Here's how the part is built. I have some questions about the finished solid (model axes, mm). Face numbers are marked on the shaded views. A direction names the side the tool comes from. Coordinates: 2 decimals unless noted, no trailing zeros. Write each loop counter-clockwise with the first axis right and the second up, starting at its lowest first coordinate (ties: lowest second). Pieces come first, ordered by that corner, then holes.
Item 1: If I drill on line 1 (Y direction, x = 17.2, z = 0); line 2 (Y direction, x = 0, z = -30.25) (3 decimals), over which ranges is the centre line in solid material (lowest first)?
Item 2: If we section it at A-A (z = 0): Count the separate pieces of the cut face and the enclosed holes in it, then the cut area to 3 significant figures.
Item 3: If we section it at B-B (x = 0): Please give me the cut outline in (y, z) (3 decimals), then the cut area to 3 significant figures.
Item 4: For the marked faces 4, 5 and 6, which set-ups out of +Z, -Z, +X, -X, +Y, -Y let a thin tool reach every point of the face, with its end or its side?
Item 5: I'm going to push flat-ended pins straight in: pin 1 Ø8 at (x, z) = (14, -14) entering from -Y; pin 2 Ø12 at (y, z) = (9, -8) entering from -X; pin 3 Ø7.5 at (x, y) = (-0.5, -9) entering from +Z; pin 4 Ø5 at (x, z) = (14.5, -6) entering from +Y. Where does each tip first touch, or does it pass through?
Item 6: We'd pull the mould along Z, two halves only. Please class the marked faces 1, 2 and 3: +Z half, -Z half, draft (parallel to the pull), parting line (faces both ways), or undercut.
from build123d import *

# Parameters (mm, degrees)
BOSS_EXTRUDE1_DEPTH             = 10
CUT_EXTRUDE1_DEPTH              = 46.82575695
CUT_EXTRUDE1_DEPTH_BACK         = 46.82575695
SKETCH2_R                       = 7.5
SKETCH3_R                       = 12.7
SKETCH3_R_2                     = 9.525
BOSS_EXTRUDE2_DEPTH             = 20
BOSS_EXTRUDE2_DIRECTION_2_REACH = 41.449
CUT_EXTRUDE2_DEPTH              = 41.21865247
CUT_EXTRUDE2_DEPTH_BACK         = 41.21865247
FILLET1_R                       = 10
FILLET2_R                       = 2.5


with BuildPart() as part:
    # Sketch1 → Boss-Extrude1 (new, symmetric)
    with BuildSketch(Plane(origin=(0, 0, 0), x_dir=(1, 0, 0), z_dir=(0, 1, 0))):
        with BuildLine():
            Line((-20, 7.5), (-20, 0))
            Line((-20, 0), (-15, 0))
            Line((-15, 0), (-15, 7.5))
            ThreePointArc((-15, 7.5), (-12.803300859, 12.803300859), (-7.5, 15))
            Line((-7.5, 15), (7.5, 15))
            ThreePointArc((7.5, 15), (12.803300859, 12.803300859), (15, 7.5))
            Line((15, 7.5), (15, 0))
            Line((15, 0), (20, 0))
            Line((20, 0), (20, 7.5))
            ThreePointArc((20, 7.5), (16.338834765, 16.338834765), (7.5, 20))
            Line((7.5, 20), (-7.5, 20))
            ThreePointArc((-7.5, 20), (-16.338834765, 16.338834765), (-20, 7.5))
        make_face()
        Polygon((-15, 0), (-20, 0), (-20, -7.5), (-20, -12.5), (-15, -12.5), (-15, -7.5), align=None)
        Polygon((20, 0), (15, 0), (15, -7.5), (15, -12.5), (20, -12.5), (20, -7.5), align=None)
    extrude(amount=BOSS_EXTRUDE1_DEPTH, both=True)

    # Sketch2 → Cut-Extrude1 (cut, two sides: drawn at the far end of the back side and taken through both)
    with BuildSketch(Plane(origin=(20, 0, 0), x_dir=(0, 0, -1), z_dir=(1, 0, 0)).offset(-CUT_EXTRUDE1_DEPTH_BACK)):
        Circle(SKETCH2_R)
    extrude(amount=CUT_EXTRUDE1_DEPTH + CUT_EXTRUDE1_DEPTH_BACK, mode=Mode.SUBTRACT)

    # Sketch3 → Boss-Extrude2 (add)
    with BuildSketch(Plane(origin=(0, 0, -20), x_dir=(-1, 0, 0), z_dir=(0, 0, -1))):
        Circle(SKETCH3_R)
        Circle(SKETCH3_R_2, mode=Mode.SUBTRACT)
    extrude(amount=BOSS_EXTRUDE2_DEPTH)

    # Boss-Extrude2 direction 2: up to this face of the body (flat: up to its plane)
    boss_extrude2_direction_2_end = Plane(part.part.faces().sort_by_distance((0, 0, -15))[0])
    # Sketch3 → Boss-Extrude2 direction 2 (add, up to the picked face)
    with BuildSketch(Plane(origin=(0, 0, -20), x_dir=(-1, 0, 0), z_dir=(0, 0, -1)), mode=Mode.PRIVATE) as boss_extrude2_direction_2_sk1:
        Circle(SKETCH3_R)
        Circle(SKETCH3_R_2, mode=Mode.SUBTRACT)
    boss_extrude2_direction_2_tool1 = split(extrude(boss_extrude2_direction_2_sk1.sketch, amount=-BOSS_EXTRUDE2_DIRECTION_2_REACH, mode=Mode.PRIVATE), bisect_by=boss_extrude2_direction_2_end, keep=Keep.BOTH, mode=Mode.PRIVATE)
    add(boss_extrude2_direction_2_tool1.solids().sort_by(Axis((12.34079, 0, -20), (0, 0, 1)))[0])

    # Sketch3<2> → Cut-Extrude2 (cut, two sides: drawn at the far end of the back side and taken through both)
    with BuildSketch(Plane(origin=(0, 0, -20), x_dir=(-1, 0, 0), z_dir=(0, 0, -1)).offset(-CUT_EXTRUDE2_DEPTH_BACK)):
        with BuildLine():
            Line((7.5, -5.871594758), (7.5, 5.871594758))
            ThreePointArc((7.5, 5.871594758), (0, 9.525), (-7.5, 5.871594758))
            Line((-7.5, 5.871594758), (-7.5, -5.871594758))
            ThreePointArc((-7.5, -5.871594758), (0, -9.525), (7.5, -5.871594758))
        make_face()
        with BuildLine():
            Line((-7.5, -5.871594758), (-7.5, 5.871594758))
            ThreePointArc((-7.5, 5.871594758), (-9.525, 0), (-7.5, -5.871594758))
        make_face()
        with BuildLine():
            ThreePointArc((7.5, -5.871594758), (9.00453011, -3.105489092), (9.525, 0))
            ThreePointArc((9.525, 0), (9.00453011, 3.105489092), (7.5, 5.871594758))
            Line((7.5, 5.871594758), (7.5, -5.871594758))
        make_face()
    extrude(amount=CUT_EXTRUDE2_DEPTH + CUT_EXTRUDE2_DEPTH_BACK, mode=Mode.SUBTRACT)

    # Fillet1
    fillet1_edges = [part.edges().sort_by_distance(p)[0] for p in [
        (17.5, -10, 12.5),
        (-17.5, -10, 12.5),
        (-17.5, 10, 12.5),
        (17.5, 10, 12.5),
    ]]
    fillet(fillet1_edges, radius=FILLET1_R - 0.0001)  # a hair under: the kernel refuses the full size

    # Fillet2
    fillet2_edges = [part.edges().sort_by_distance(p)[0] for p in [
        (20, 10, -2.49995),
        (-20, -10, -2.49995),
        (-20, 10, -2.49995),
        (-20, 7.071097101, 9.571097101),
        (-20, -7.071097101, 9.571097101),
        (16.454326123, -10, -16.221814243),
        (-16.454326123, -10, -16.221814243),
        (-16.454326123, 10, -16.221814243),
        (16.454326123, 10, -16.221814243),
        (20, -10, -2.49995),
        (20, 7.071097101, 9.571097101),
    ]]
    fillet(fillet2_edges, radius=FILLET2_R - 0.0001)  # a hair under: the kernel refuses the full size


solid = part.part
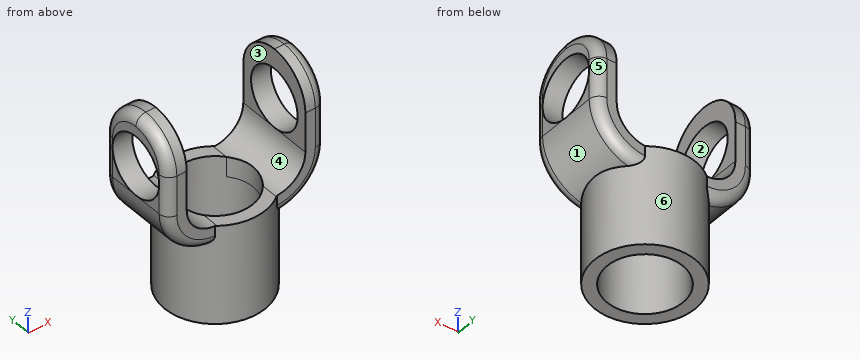
Answer list:
1. line 1: y = -10 to -7.5, 7.5 to 10
1. line 2: y = -12.7 to -9.525, 9.525 to 12.7
2. separate pieces: 4
2. enclosed holes: 0
2. area: 44.6 mm2
3. outline: (-12.7, -40) - (-9.525, -40) - (-9.525, -15) - (-12.7, -15) - close; (9.525, -40) - (12.7, -40) - (12.7, -15) - (9.525, -15) - close
3. area: 159 mm2
4. face 4: +Z, +Y, -Y
4. face 5: +Z, -Z, +X, +Y
4. face 6: -Z
5. pin 1: stops at y = -10
5. pin 2: stops at x = -20
5. pin 3: stops at z = -15
5. pin 4: stops at y = 10
6. face 1: -Z half
6. face 2: undercut
6. face 3: draft
